The model under review builds one solid part; all positions refer to its coordinate system, in mm. Face numbers are marked on the shaded views. A direction names the side the tool comes from. Coordinates: 2 decimals unless noted, no trailing zeros. Write each loop counter-clockwise with the first axis right and the second up, starting at its lowest first coordinate (ties: lowest second). Pieces come first, ordered by that corner, then holes.
```python
from build123d import *

# Parameters (mm, degrees)
BOSS_EXTRUDE1_DEPTH = 3.81
BOSS_EXTRUDE2_DEPTH = 8.255
SKETCH3_W           = 64.77
SKETCH3_H           = 7.1
CUT_EXTRUDE1_DEPTH  = 0.635
CUT_EXTRUDE4_DEPTH  = 4.81
CUT_EXTRUDE5_DEPTH  = 4.81
SKETCH12_R          = 2.4257
CUT_EXTRUDE6_DEPTH  = 4.81
SKETCH4_R           = 1.143
CUT_EXTRUDE2_DEPTH  = 11.43
SKETCH17_R          = 2.413
CUT_EXTRUDE9_DEPTH  = 4.81
BOSS_EXTRUDE5_DEPTH = 8.255
SKETCH20_W          = 69.85
SKETCH20_H          = 3.175
BOSS_EXTRUDE6_DEPTH = 2.54
SKETCH21_R          = 1.02235
CUT_EXTRUDE10_DEPTH = 13.065


with BuildPart() as part:
    # Sketch1 → Boss-Extrude1 (new body)
    with BuildSketch(Plane.XY):
        with BuildLine():
            Line((10.977415053, 19.05), (44.196, 19.05))
            ThreePointArc((44.196, 19.05), (48.686128061, 20.909871939), (50.546, 25.4))
            Line((50.546, 25.4), (50.546, 44.45))
            Line((50.546, 44.45), (61.579155694, 44.45))
            ThreePointArc((61.579155694, 44.45), (75.946, 0), (61.579155694, -44.45))
            Line((61.579155694, -44.45), (50.546, -44.45))
            Line((50.546, -44.45), (50.546, -25.4))
            ThreePointArc((50.546, -25.4), (48.686128061, -20.909871939), (44.196, -19.05))
            Line((44.196, -19.05), (10.977415053, -19.05))
            ThreePointArc((10.977415053, -19.05), (6.487286992, -20.909871939), (4.627415053, -25.4))
            Line((4.627415053, -25.4), (-71.572584947, -25.4))
            ThreePointArc((-71.572584947, -25.4), (-75.946, 0), (-71.572584947, 25.4))
            Line((-71.572584947, 25.4), (4.627415053, 25.4))
            ThreePointArc((4.627415053, 25.4), (6.487286992, 20.909871939), (10.977415053, 19.05))
        make_face()
    extrude(amount=BOSS_EXTRUDE1_DEPTH)

    # Sketch2 → Boss-Extrude2 (add)
    with BuildSketch(Plane.XY.offset(3.81)):
        with BuildLine():
            Line((61.865268471, 17.78), (60.095110466, 38.1))
            ThreePointArc((60.095110466, 38.1), (59.464196764, 40.158289632), (58.047089349, 41.778911391))
            Line((58.047089349, 41.778911391), (57.900800643, 44.704))
            Line((57.900800643, 44.704), (61.395010384, 44.704))
            ThreePointArc((61.395010384, 44.704), (69.822038137, 29.877715884), (74.728381149, 13.544887112))
            Line((74.728381149, 13.544887112), (60.759450402, 13.544887112))
            Line((60.759450402, 13.544887112), (60.759450402, 15.094127876))
            ThreePointArc((60.759450402, 15.094127876), (61.639191639, 16.302501703), (61.865268471, 17.78))
        make_face()
        with BuildLine():
            Line((58.651639318, 17.500047669), (56.881481313, 37.820047669))
            Line((56.881481313, 37.820047669), (50.546, 37.820047669))
            Line((50.546, 37.820047669), (50.546, 16.566735288))
            Line((50.546, 16.566735288), (57.366094516, 16.566735288))
            ThreePointArc((57.366094516, 16.566735288), (58.160401987, 16.824667019), (58.651639318, 17.500047669))
        make_face()
        with BuildLine():
            Line((60.759450402, -13.544887112), (74.728381149, -13.544887112))
            ThreePointArc((74.728381149, -13.544887112), (69.822038137, -29.877715884), (61.395010384, -44.704))
            Line((61.395010384, -44.704), (57.900800643, -44.704))
            Line((57.900800643, -44.704), (58.047089349, -41.778911391))
            ThreePointArc((58.047089349, -41.778911391), (59.464196764, -40.158289632), (60.095110466, -38.1))
            Line((60.095110466, -38.1), (61.865268471, -17.78))
            ThreePointArc((61.865268471, -17.78), (61.639191639, -16.302501703), (60.759450402, -15.094127876))
            Line((60.759450402, -15.094127876), (60.759450402, -13.544887112))
        make_face()
        with BuildLine():
            Line((50.546, -16.566735288), (57.366094516, -16.566735288))
            ThreePointArc((57.366094516, -16.566735288), (58.160401987, -16.824667019), (58.651639318, -17.500047669))
            Line((58.651639318, -17.500047669), (56.881481313, -37.820047669))
            Line((56.881481313, -37.820047669), (50.546, -37.820047669))
            Line((50.546, -37.820047669), (50.546, -16.566735288))
        make_face()
    extrude(amount=BOSS_EXTRUDE2_DEPTH)

    # Sketch3 → Cut-Extrude1 (cut)
    with BuildSketch(Plane.XY.offset(3.81)):
        with Locations((44.577, 0)):
            Rectangle(SKETCH3_W, SKETCH3_H)
    extrude(amount=-CUT_EXTRUDE1_DEPTH, mode=Mode.SUBTRACT)

    # Sketch9 → Cut-Extrude4 (cut, through all)
    with BuildSketch(Plane.XY.offset(3.81)):
        with BuildLine():
            Line((69.85, 11.17), (25.4, 11.17))
            ThreePointArc((25.4, 11.17), (21.971, 7.741), (25.4, 4.312))
            Line((25.4, 4.312), (69.85, 4.312))
            ThreePointArc((69.85, 4.312), (73.279, 7.741), (69.85, 11.17))
        make_face()
        with BuildLine():
            Line((69.85, -4.312), (25.4, -4.312))
            ThreePointArc((25.4, -4.312), (21.971, -7.741), (25.4, -11.17))
            Line((25.4, -11.17), (69.85, -11.17))
            ThreePointArc((69.85, -11.17), (73.279, -7.741), (69.85, -4.312))
        make_face()
    extrude(amount=-CUT_EXTRUDE4_DEPTH, mode=Mode.SUBTRACT)

    # Sketch10 → Cut-Extrude5 (cut, through all)
    with BuildSketch(Plane.XY.offset(3.81)):
        with BuildLine():
            Line((-10.922, 11.43), (-59.182, 11.43))
            ThreePointArc((-59.182, 11.43), (-61.42706403, 10.50006403), (-62.357, 8.255))
            Line((-62.357, 8.255), (-62.357, -8.255))
            ThreePointArc((-62.357, -8.255), (-61.42706403, -10.50006403), (-59.182, -11.43))
            Line((-59.182, -11.43), (-10.922, -11.43))
            ThreePointArc((-10.922, -11.43), (-8.67693597, -10.50006403), (-7.747, -8.255))
            Line((-7.747, -8.255), (-7.747, 8.255))
            ThreePointArc((-7.747, 8.255), (-8.67693597, 10.50006403), (-10.922, 11.43))
        make_face()
    extrude(amount=-CUT_EXTRUDE5_DEPTH, mode=Mode.SUBTRACT)

    # Sketch12 → Cut-Extrude6 (cut, through all)
    with BuildSketch(Plane.XY.offset(3.81)):
        with Locations((15.24, 11.43)):
            Circle(SKETCH12_R)
        with Locations((15.24, -11.43)):
            Circle(SKETCH12_R)
    extrude(amount=-CUT_EXTRUDE6_DEPTH, mode=Mode.SUBTRACT)

    # Sketch4 → Cut-Extrude2 (cut)
    with BuildSketch(Plane.XY.offset(3.175)):
        with Locations((19.812, 0)):
            Circle(SKETCH4_R)
        with Locations((34.798, 0)):
            Circle(SKETCH4_R)
        with Locations((49.784, 0)):
            Circle(SKETCH4_R)
        with Locations((64.77, 0)):
            Circle(SKETCH4_R)
    extrude(amount=-CUT_EXTRUDE2_DEPTH, mode=Mode.SUBTRACT)

    # Sketch17 → Cut-Extrude9 (cut, through all)
    with BuildSketch(Plane.XY.offset(3.81)):
        with Locations((-0.127, 16.51)):
            Circle(SKETCH17_R)
        with Locations((-0.127, -16.51)):
            Circle(SKETCH17_R)
    extrude(amount=-CUT_EXTRUDE9_DEPTH, mode=Mode.SUBTRACT)

    # Sketch19 → Boss-Extrude5 (add)
    with BuildSketch(Plane.XY.offset(3.81)):
        with BuildLine():
            Line((-71.572584947, -25.4), (-65.222584947, -25.4))
            Line((-65.222584947, -25.4), (-65.222584947, 25.4))
            Line((-65.222584947, 25.4), (-71.572584947, 25.4))
            ThreePointArc((-71.572584947, 25.4), (-75.946, 0), (-71.572584947, -25.4))
        make_face()
    extrude(amount=BOSS_EXTRUDE5_DEPTH)

    # Sketch20 → Boss-Extrude6 (add)
    with BuildSketch(Plane.XZ.offset(25.4)):
        with Locations((-30.297584947, 5.3975)):
            Rectangle(SKETCH20_W, SKETCH20_H)
    boss_extrude6 = extrude(amount=-BOSS_EXTRUDE6_DEPTH)

    # Mirror1: Boss-Extrude6 across plane
    add(boss_extrude6.mirror(Plane.ZX))

    # Sketch21 → Cut-Extrude10 (cut, through all)
    with BuildSketch(Plane(origin=(0, 0, 0), x_dir=(-1, 0, 0), z_dir=(0, 0, -1))):
        with Locations((54.102, 19.05)):
            Circle(SKETCH21_R)
        with Locations((16.002, 19.05)):
            Circle(SKETCH21_R)
        with Locations((16.002, -19.05)):
            Circle(SKETCH21_R)
        with Locations((54.102, -19.05)):
            Circle(SKETCH21_R)
    extrude(amount=-CUT_EXTRUDE10_DEPTH, mode=Mode.SUBTRACT)


solid = part.part
```
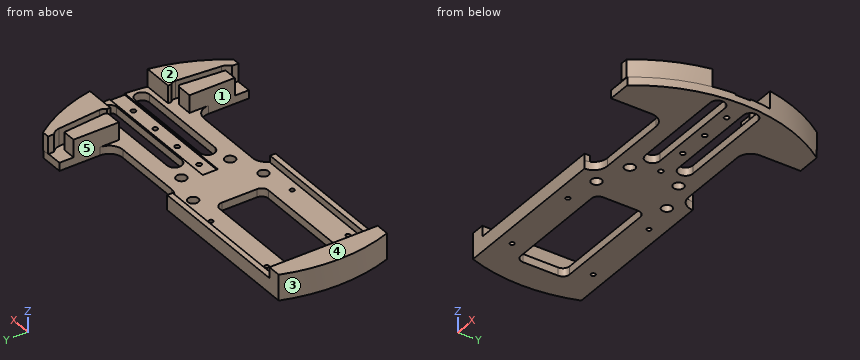
Item 1: Take a section at D-D, the plane x = 15.24. Write out the cut boundary in (y, z) (3 decimals), plus the area to 3 significant figures.
Solved:
outline: (-19.05, 0) - (-13.856, 0) - (-13.856, 3.81) - (-19.05, 3.81) - close; (-9.004, 0) - (9.004, 0) - (9.004, 3.81) - (3.55, 3.81) - (3.55, 3.175) - (-3.55, 3.175) - (-3.55, 3.81) - (-9.004, 3.81) - close; (13.856, 0) - (19.05, 0) - (19.05, 3.81) - (13.856, 3.81) - close
area: 104 mm2
Item 2: For pin 1 (6 mm diameter, centred on x = 31.5, z = 8.5, fed in from -Y); pin 2 (6 mm diameter, centred on y = 8.5, z = 3.5, fed in from +X); pin 3 (3 mm diameter, centred on y = -3, z = 1.5, fed in from +X); pin 4 (1.9 mm diameter, centred on x = 38, z = 2.5, fed in from +Y), all flat-tipped, find the tip position at first contact; note any pin that passes through.
Solved:
pin 1: passes through
pin 2: stops at x = 75.75
pin 3: stops at x = 75.93
pin 4: stops at y = 19.05
Item 3: Mouldability with a two-part tool opening along X and no side actions: class the marked faces 1, 2 and 3 as pulls with the +X half, pulls with the -X half, needs draft (parallel to the pull), parting line crosses it, or undercut.
Solved:
face 1: undercut
face 2: needs draft
face 3: pulls with the -X half
Item 4: To check wall thickness, follow line 1 along Y through (x, z) = (-59.5, 1); line 2 along X through (y, z) = (-20, 11); line 3 along Y through (x, z) = (53.5, 6.5). State the ranges of each line that lie inside material, in increasing order.
Solved:
line 1: y = -25.4 to -11.41, 11.41 to 25.4
line 2: x = -73.27 to -65.22, 50.55 to 58.43, 61.67 to 73.27
line 3: y = -37.82 to -16.57, 16.57 to 37.82
Item 5: Take a section at B-B, the plane x = -57.5. Write out the cut boundary in (y, z) (3 decimals), plus the area to 3 significant figures.
Solved:
outline: (-25.4, 0) - (-11.43, 0) - (-11.43, 3.81) - (-22.86, 3.81) - (-22.86, 6.985) - (-25.4, 6.985) - close; (11.43, 0) - (25.4, 0) - (25.4, 6.985) - (22.86, 6.985) - (22.86, 3.81) - (11.43, 3.81) - close
area: 123 mm2
Item 6: Take a section at C-C, the plane z = 10. Count the separate pieces of the cut face and the enclosed holes in it, plus the area to 3 significant figures.
Solved:
separate pieces: 5
enclosed holes: 0
area: 1,330 mm2
Item 7: Take a section at A-A, the plane x = 31. Write out the cut boundary in (y, z) (3 decimals).
Solved:
outline: (-19.05, 0) - (-11.17, 0) - (-11.17, 3.81) - (-19.05, 3.81) - close; (-4.312, 0) - (4.312, 0) - (4.312, 3.81) - (3.55, 3.81) - (3.55, 3.175) - (-3.55, 3.175) - (-3.55, 3.81) - (-4.312, 3.81) - close; (11.17, 0) - (19.05, 0) - (19.05, 3.81) - (11.17, 3.81) - close
Item 8: Machinability: for the marked faces 4 and 5, which of the approach directions +Z, -Z, +X, -X, +Y, -Y give a long, thin tool a straight path to every point of the face, cutting with its end or side? Answer none if there is none.
Solved:
face 4: +Z, +X, -X, +Y, -Y
face 5: +Z, +Y
